Autodesk Inventor part; units mm, degrees
ref_plane "YZ Plane" through (0, 0, 0) normal (1, 0, 0) x (0, 1, 0)
ref_plane "XZ Plane" through (0, 0, 0) normal (0, 1, 0) x (-1, 0, 0)
ref_plane "XY Plane" through (0, 0, 0) normal (0, 0, 1) x (1, 0, 0)
sketch "Sketch1" plane through (0, 0, 0) normal (0, 1, 0) x (-1, 0, 0)
  line L0 (-28.5, 28.5) -> (28.5, 28.5)
  line L1 (28.5, 28.5) -> (28.5, -28.5)
  line L2 (28.5, -28.5) -> (-28.5, -28.5)
  line L3 (-28.5, -28.5) -> (-28.5, 28.5)
  line L4 (-28.5, 28.5) -> (28.5, -28.5) construction
  line L5 (28.5, 28.5) -> (-28.5, -28.5) construction
  point P0 (0, 0)
  dimension "d0" = 57
  dimension "d1" = 57
extrude "Extrusion1" add sketch "Sketch1" along normal blind 56
sketch "Sketch2" plane through (0, 56, 0) normal (0, 1, 0) x (1, 0, 0)
  circle A0 centre (-23.57, 23.57) radius 2.6
  point P0 (0, 0)
  dimension "d6" = 5.2
  dimension "d19" = 23.57
  dimension "d20" = 23.57
extrude "Extrusion2" cut sketch "Sketch2" against normal blind 4.8
pattern_linear "Rectangular Pattern1" count 2 spacing 47.14 along (1, 0, 0) count 2 spacing 47.14 along (0, 0, 1) of "Extrusion2"
fillet "Fillet1" radius 4 4 edges at (28.5, 28, -28.5) (-28.5, 28, -28.5) (28.5, 28, 28.5) (-28.5, 28, 28.5)
sketch "Sketch3" plane through (0, 56, 0) normal (0, 1, 0) x (1, 0, 0)
  circle A0 centre (0, 0) radius 3.175
  dimension "d16" = 6.35
extrude "Extrusion3" add sketch "Sketch3" along normal blind 26
properties part number "Motor Nema23"
Can you work these out from the model? Positions are in its coordinate system, mm. A direction names the side the tool comes from. Give positions to 0.01 mm unless a question says otherwise; leave off trailing zeros. Loops run counter-clockwise (first coordinate to the right, second up) from the corner with the lowest first, then second, coordinate; pieces in that order, holes last. Notation, with made-up numbers: (64.5, 84.5) - (119.5, 84.5) arc R19 ccw to (119.5, 119.5) - close; hole circle Ø7 at (43.5, 44). An arc over 180 degrees is marked (long way). Return JSON: item names as keys, results as strings.
1. I'm going to push flat-ended pins straight in: pin 1 Ø4 at (x, z) = (24.5, -23) entering from +Y; pin 2 Ø2.5 at (x, z) = (-22.5, 23) entering from +Y. Where does each tip first touch, or does it pass through?
Output values:
{"pin 1": "stops at y = 56", "pin 2": "stops at y = 51.2"}
2. I want a section at D-D on x = 0. Please give me the cut outline in (y, z) (3 decimals), and give its area (3 significant figures).
Output values:
{"outline": "(0, -28.5) - (56, -28.5) - (56, -3.175) - (82, -3.175) - (82, 3.175) - (56, 3.175) - (56, 28.5) - (0, 28.5) - close", "area": "3,360 mm²"}
3. I want a section at C-C on y = 73. Please give me the cut outline in (x, z) (3 decimals), and give its area (3 significant figures).
Output values:
{"outline": "circle Ø6.35 at (0, 0)", "area": "31.7 mm²"}
4. We'd pull the mould along Z, two halves only. Please class faces 1 (the face through (-24, 51.2, -24)), 2 (the face through (28.5, 28, 0)), 3 (the face through (-24, 51.2, 24)), 4 (the face through (0, 28, -28.5)): +Z half, -Z half, draft (parallel to the pull), parting line (faces both ways), or undercut.
Output values:
{"face 1": "undercut", "face 2": "draft", "face 3": "undercut", "face 4": "-Z half"}
5. If I drill on line 1 (X direction, y = 54.8, z = 23.57); line 2 (Z direction, x = 23, y = 53), over which ranges is the centre line in solid material (lowest first)?
Output values:
{"line 1": "x = -28.5 to -26.17, -20.97 to 20.97, 26.17 to 28.5", "line 2": "z = -28.5 to -26.11, -21.03 to 21.03, 26.11 to 28.5"}
6. For faces 5 (the face through (24, 51.2, -24)), 6 (the face through (-27.297, 28.392, -27.359)), which set-ups out of +Z, -Z, +X, -X, +Y, -Y let a thin tool reach every point of the face, with its end or its side?
Output values:
{"face 5": "+Y", "face 6": "-Z, -X, +Y, -Y"}
7. I want a section at B-B on z = 0. Please give me the cut outline in (x, y) (3 decimals), and give its area (3 significant figures).
Output values:
{"outline": "(-28.5, 0) - (28.5, 0) - (28.5, 56) - (3.175, 56) - (3.175, 82) - (-3.175, 82) - (-3.175, 56) - (-28.5, 56) - close", "area": "3,360 mm²"}
8. I want a section at A-A on x = 23.57. Please give me the cut outline in (y, z).
Output values:
{"outline": "(0, -28.5) - (56, -28.5) - (56, -26.17) - (51.2, -26.17) - (51.2, -20.97) - (56, -20.97) - (56, 20.97) - (51.2, 20.97) - (51.2, 26.17) - (56, 26.17) - (56, 28.5) - (0, 28.5) - close"}
